from build123d import *

# Parameters (mm, degrees)
PLATE_DEPTH           = 4
SKETCH2_R             = 1.5
PLATE_MOUNTINGS_DEPTH = 130.631207662
SKETCH3_R             = 1.5
SKETCH3_R_2           = 2.31
SKETCH3_R_3           = 9.25
SKETCH3_W             = 11.5
SKETCH3_H             = 22
CUT_EXTRUDE1_DEPTH    = 130.631207662
SKETCH4_R             = 1.59
CUT_EXTRUDE2_DEPTH    = 130.631207662


with BuildPart() as part:
    # Sketch1 → Plate (new body)
    with BuildSketch(Plane(origin=(0, 0, 0), x_dir=(1, 0, 0), z_dir=(0, 1, 0))):
        with BuildLine():
            Line((62, 4), (46.5, 4))
            Line((46.5, 4), (46.5, 75.5))
            Line((46.5, 75.5), (66, 75.5))
            ThreePointArc((66, 75.5), (0, 111.5), (-66, 75.5))
            Line((-66, 75.5), (-46.5, 75.5))
            Line((-46.5, 75.5), (-46.5, 4))
            Line((-46.5, 4), (-62, 4))
            ThreePointArc((-62, 4), (-66, 0), (-62, -4))
            Line((-62, -4), (-46.5, -4))
            Line((-46.5, -4), (-46.5, -75.5))
            Line((-46.5, -75.5), (-66, -75.5))
            ThreePointArc((-66, -75.5), (0, -111.5), (66, -75.5))
            Line((66, -75.5), (46.5, -75.5))
            Line((46.5, -75.5), (46.5, -4))
            Line((46.5, -4), (62, -4))
            ThreePointArc((62, -4), (66, 0), (62, 4))
        make_face()
    extrude(amount=PLATE_DEPTH)

    # Sketch2 → Plate mountings (cut, through all)
    with BuildSketch(Plane(origin=(0, 4, 0), x_dir=(1, 0, 0), z_dir=(0, 1, 0))):
        with Locations(Location((55, 0, 0), (0, 0, 270))):
            Circle(SKETCH2_R)
        with Locations(Location((55, 80, 0), (0, 0, 270))):
            Circle(SKETCH2_R)
        with Locations(Location((-55, 0, 0), (0, 0, 90))):
            Circle(SKETCH2_R)
        with Locations(Location((-55, 80, 0), (0, 0, 90))):
            Circle(SKETCH2_R)
        with Locations(Location((52.5, -84, 0), (0, 0, 270))):
            Circle(SKETCH2_R)
        with Locations(Location((-52.5, -84, 0), (0, 0, 90))):
            Circle(SKETCH2_R)
    extrude(amount=-PLATE_MOUNTINGS_DEPTH, mode=Mode.SUBTRACT)

    # Sketch3 → Cut-Extrude1 (cut, through all)
    with BuildSketch(Plane(origin=(0, 4, 0), x_dir=(1, 0, 0), z_dir=(0, 1, 0))):
        with Locations(Location((-16.75, -98.5, 0), (0, 0, 270))):
            Circle(SKETCH3_R)
        with Locations(Location((1.5, -69.5, 0), (0, 0, 270))):
            Circle(SKETCH3_R_2)
        with Locations(Location((1.5, -97.5, 0), (0, 0, 90))):
            Circle(SKETCH3_R_2)
        with Locations(Location((-16.75, -83.5, 0), (0, 0, 270))):
            Circle(SKETCH3_R)
        with Locations(Location((-16.75, -68.5, 0), (0, 0, 270))):
            Circle(SKETCH3_R)
        with Locations(Location((0, -51.5, 0), (0, 0, 270))):
            Circle(SKETCH3_R_3)
        with Locations((1.5, -83.5)):
            Rectangle(SKETCH3_W, SKETCH3_H)
    extrude(amount=-CUT_EXTRUDE1_DEPTH, mode=Mode.SUBTRACT)

    # Sketch4 → Cut-Extrude2 (cut, through all)
    with BuildSketch(Plane(origin=(0, 4, 0), x_dir=(1, 0, 0), z_dir=(0, 1, 0))):
        with Locations(Location((18.11, 9.96, 0), (0, 0, 270))):
            Circle(SKETCH4_R)
        with Locations(Location((-33.96, 4.88, 0), (0, 0, 270))):
            Circle(SKETCH4_R)
        with Locations(Location((-33.96, -23.06, 0), (0, 0, 270))):
            Circle(SKETCH4_R)
    extrude(amount=-CUT_EXTRUDE2_DEPTH, mode=Mode.SUBTRACT)


solid = part.part
Design review of the part built by this model. Coordinates are the model's own, in mm. A direction names the side the tool comes from. Give positions to 0.01 mm unless a question says otherwise; leave off trailing zeros. Write each loop counter-clockwise with the first axis right and the second up, starting at its lowest first coordinate (ties: lowest second). Pieces come first, ordered by that corner, then holes. Notation, with made-up numbers: M 43,-22 L 94,-22 A23 cw 94,-9 Z; hole C 39,44.5 d8. An arc over 180 degrees is marked long. Return JSON: item names as keys, results as strings. Group by question number.
Item 1: Take a section at B-B (z = 78.5). Give the boundary of the cut face in (x, y).
Item 2: Tool access review of faces 4 (the flat face through (46.5, 2, -39)), 5 (the flat face through (-4.25, 2, 84)), 6 (the flat face through (-56, 2, -75.5)): name each direction out of +Z, -Z, +X, -X, +Y, -Y from which nothing blocks a thin tool from reaching the whole face with its end or side.
Item 3: The part is to be moulded in two halves that separate along X. For faces 1 (the cylindrical face through (1.098, 1.972, -111.492)), 2 (the flat face through (1, 2, 94.5)), 3 (the flat face through (46.5, 2, 40)), say which applies: pulls with the +X half, pulls with the -X half, needs draft (parallel to the pull), parting line crosses it, or undercut.
Item 4: Clearance check with flat-ended pins moving along their axes: pin 1 Ø1.2 at (x, y) = (51, 2) entering from +Z; pin 2 Ø2 at (x, y) = (52, 3) entering from -Z; pin 3 Ø2 at (x, y) = (-50.5, 2.5) entering from -Z. State where each tip first meets the part, or that it passes through.
Item 5: Take a section at C-C (y = 1.3). Count the separate pieces of the cut face and the enclosed holes in it, plus the area to 3 significant figures.
Item 6: Wall thickness on line 1 along X through (y, z) = (2.15, 0); line 2 along X through (y, z) = (1.45, 84); line 3 along X through (y, z) = (2.8, -80): over which ranges is each line inside the solid? List them lowest first.
Item 7: Take a section at A-A (z = 51.5). Give the boundary of the cut face in (x, y), plus the area to 3 significant figures.
Item 8: Take a section at D-D (z = -66.5). Give the boundary of the cut face in (x, y).
Return value:
{
 "1": {"outline": "M -63.97,0 L -4.25,0 L -4.25,4 L -63.97,4 Z; M 7.25,0 L 63.97,0 L 63.97,4 L 7.25,4 Z"},
 "2": {"face 4": "+X, +Y, -Y", "face 5": "+Y, -Y", "face 6": "-X, +Y, -Y"},
 "3": {"face 1": "parting line crosses it", "face 2": "undercut", "face 3": "pulls with the +X half"},
 "4": {"pin 1": "stops at z = 93.18", "pin 2": "stops at z = -92.68", "pin 3": "stops at z = -93.93"},
 "5": {"separate pieces": "1", "enclosed holes": "16", "area": "20,400 mm2"},
 "6": {"line 1": "x = -66 to -56.5, -53.5 to 53.5, 56.5 to 66", "line 2": "x = -59.68 to -54, -51 to -18.16, -15.34 to -4.25, 7.25 to 51, 54 to 59.68", "line 3": "x = -62.87 to -56.5, -53.5 to 53.5, 56.5 to 62.87"},
 "7": {"outline": "M -46.5,0 L -9.25,0 L -9.25,4 L -46.5,4 Z; M 9.25,0 L 46.5,0 L 46.5,4 L 9.25,4 Z", "area": "298 mm2"},
 "8": {"outline": "M -46.5,0 L 46.5,0 L 46.5,4 L -46.5,4 Z"}
}
